Read the model definition and answer for the solid it produces. Units are mm, in the model's axes. A direction names the side the tool comes from. Round coordinates to 2 decimals unless told otherwise and drop trailing zeros. Loops run counter-clockwise (first coordinate to the right, second up) from the corner with the lowest first, then second, coordinate; pieces in that order, holes last. Notation, with made-up numbers: M 59.5,-9.75 L 88.5,-9.75 A9 ccw 88.5,5.25 Z; hole C -34.75,37.5 d4. An arc over 180 degrees is marked long. Write each question's results on one line, items separated by ' | '.
from build123d import *

# Parameters (mm, degrees)
PAD_DEPTH            = 2
PAD001_DEPTH         = 3.5
SKETCH002_R          = 1.5
POCKET_DEPTH         = 5
POCKET001_DEPTH      = 5
LINEARPATTERN_COUNT  = 12
LINEARPATTERN_PITCH  = 4.545455
SKETCH004_W          = 12
SKETCH004_H          = 7.5
POCKET002_DEPTH      = 10
POCKET002_DEPTH_BACK = -100


with BuildPart() as part:
    # Sketch → Pad (new body)
    with BuildSketch(Plane.XY):
        with BuildLine():
            Line((-44.5, 38), (44.5, 38))
            ThreePointArc((49.5, 33), (48.035534, 36.535534), (44.5, 38))
            Line((49.5, 33), (49.5, -33))
            ThreePointArc((44.5, -38), (48.035534, -36.535534), (49.5, -33))
            Line((44.5, -38), (-44.5, -38))
            ThreePointArc((-49.5, -33), (-48.035534, -36.535534), (-44.5, -38))
            Line((-49.5, -33), (-49.5, 33))
            ThreePointArc((-44.5, 38), (-48.035534, 36.535534), (-49.5, 33))
        make_face()
    extrude(amount=PAD_DEPTH)

    # Sketch001 (on Face10 of Pad) → Pad001 (join)
    with BuildSketch(Plane.XY.offset(2)):
        with BuildLine():
            Line((-44.5, 36), (30.5, 36))
            ThreePointArc((33.5, 33), (32.62132, 35.12132), (30.5, 36))
            Line((33.5, 33), (33.5, 25))
            ThreePointArc((33.5, 25), (34.37868, 22.87868), (36.5, 22))
            Line((36.5, 22), (44.5, 22))
            ThreePointArc((47.5, 19), (46.62132, 21.12132), (44.5, 22))
            Line((47.5, 19), (47.5, -33))
            ThreePointArc((44.5, -36), (46.62132, -35.12132), (47.5, -33))
            Line((44.5, -36), (-30.5, -36))
            ThreePointArc((-33.5, -33), (-32.62132, -35.12132), (-30.5, -36))
            Line((-33.5, -33), (-33.5, -25))
            ThreePointArc((-33.5, -25), (-34.37868, -22.87868), (-36.5, -22))
            Line((-36.5, -22), (-44.5, -22))
            ThreePointArc((-47.5, -19), (-46.62132, -21.12132), (-44.5, -22))
            Line((-47.5, -19), (-47.5, 33))
            ThreePointArc((-44.5, 36), (-46.62132, 35.12132), (-47.5, 33))
        make_face()
        with BuildLine():
            Line((-46, -19), (-46, 33))
            ThreePointArc((-44.5, 34.5), (-45.56066, 34.06066), (-46, 33))
            Line((-44.5, 34.5), (30.5, 34.5))
            ThreePointArc((32, 33), (31.56066, 34.06066), (30.5, 34.5))
            Line((32, 33), (32, 25))
            ThreePointArc((32, 25), (33.318019, 21.818019), (36.5, 20.5))
            Line((36.5, 20.5), (44.5, 20.5))
            ThreePointArc((46, 19), (45.56066, 20.06066), (44.5, 20.5))
            Line((46, 19), (46, -33))
            ThreePointArc((44.5, -34.5), (45.56066, -34.06066), (46, -33))
            Line((44.5, -34.5), (-30.5, -34.5))
            ThreePointArc((-32, -33), (-31.56066, -34.06066), (-30.5, -34.5))
            Line((-32, -33), (-32, -25))
            ThreePointArc((-32, -25), (-33.318019, -21.818019), (-36.5, -20.5))
            Line((-36.5, -20.5), (-44.5, -20.5))
            ThreePointArc((-46, -19), (-45.56066, -20.06066), (-44.5, -20.5))
        make_face(mode=Mode.SUBTRACT)
    extrude(amount=-PAD001_DEPTH)

    # Sketch002 (on Face5 of Pad001) → Pocket (cut)
    with BuildSketch(Plane.XY.offset(2)):
        with Locations((40.5, 29)):
            Circle(SKETCH002_R)
        with Locations((-40.5, -29)):
            Circle(SKETCH002_R)
    extrude(amount=-POCKET_DEPTH, mode=Mode.SUBTRACT)

    # Sketch003 (on Face46 of Pocket) → Pocket001 (cut)
    with BuildSketch(Plane.XY.offset(2)):
        with BuildLine():
            ThreePointArc((-24, 20), (-25, 21), (-26, 20))
            Line((-26, 20), (-26, -20))
            ThreePointArc((-26, -20), (-25, -21), (-24, -20))
            Line((-24, 20), (-24, -20))
        make_face()
    pocket001 = extrude(amount=-POCKET001_DEPTH, mode=Mode.SUBTRACT)

    # LinearPattern: Pocket001 ×12
    with Locations(*[(i * LINEARPATTERN_PITCH, 0, 0) for i in range(1, LINEARPATTERN_COUNT)]):
        add(pocket001, mode=Mode.SUBTRACT)

    # Sketch004 (on Face4 of LinearPattern) → Pocket002 (cut, two sides)
    with BuildSketch(Plane(origin=(0, 0, 0), x_dir=(1, 0, 0), z_dir=(0, 0, -1))) as pocket002_sk:
        with Locations((-43.5, -19.75)):
            Rectangle(SKETCH004_W, SKETCH004_H)
    extrude(amount=-POCKET002_DEPTH, mode=Mode.SUBTRACT)
    extrude(pocket002_sk.sketch, amount=-POCKET002_DEPTH_BACK, mode=Mode.SUBTRACT)


solid = part.part
Item 1: The part is cut by section A-A (x = 40.5). Determine the outline of the cut face in (y, z), plus the area to 4 significant figures.
Outcome:
outline: M -38,0 L -36,0 L -36,-1.5 L -34.5,-1.5 L -34.5,0 L 20.5,0 L 20.5,-1.5 L 22,-1.5 L 22,0 L 27.5,0 L 27.5,2 L -38,2 Z; M 30.5,0 L 38,0 L 38,2 L 30.5,2 Z | area: 150.5 mm2
Item 2: For faces 5 (the face through (11.2, -36.4, 0)), 6 (the face through (-5.818, 0, 1)), 7 (the face through (-37.5, 20, 1)), 8 (the face through (34.36, 22.9, -0.74)), determine the directions among +Z, -Z, +X, -X, +Y, -Y from which every point of the face is accessible in a straight line to the end or side of a thin tool.
Outcome:
face 5: -Z | face 6: +Z, -Z | face 7: +Z, -Z, -X | face 8: -Z, +X, +Y
Item 3: Flat-ended cylindrical pins translate along their axes: pin 1 (1.6 mm diameter, centred on y = 19.5, z = 1, fed in from -X); pin 2 (3.5 mm diameter, centred on x = 40.5, y = 29, fed in from -Z); pin 3 (0.8 mm diameter, centred on y = -1, z = -0.5, fed in from -X). Find the tip coordinate at first contact, or state that the pin passes through.
Outcome:
pin 1: stops at x = -37.5 | pin 2: stops at z = 0 | pin 3: stops at x = -47.5
Item 4: The part is cut by section C-C (z = 1.4). State how many separate pieces and enclosed holes the cut face has, plus the area to 3 significant figures.
Outcome:
separate pieces: 1 | enclosed holes: 14 | area: 6,400 mm2
Item 5: Straight lines are drawn through the part: line 1 (Y direction, x = 14.5, z = -0.8); line 2 (X direction, y = 2, z = -0.35); line 3 (Y direction, x = 40.5, z = 1.3). For each, find the intervals that lie inside material, in ascending order.
Outcome:
line 1: y = -36 to -34.5, 34.5 to 36 | line 2: x = -47.5 to -46, 46 to 47.5 | line 3: y = -38 to 27.5, 30.5 to 38
Item 6: The mould has two halves that part along X. Classify faces 1 (the face through (-49.5, -9, 1)), 2 (the face through (-44, 16, 1)), 3 (the face through (49.5, 0, 1)), 4 (the face through (33.283, 21.853, -0.74)): pulls with the +X half, pulls with the -X half, needs draft (parallel to the pull), parting line crosses it, or undercut.
Outcome:
face 1: pulls with the -X half | face 2: needs draft | face 3: pulls with the +X half | face 4: undercut
Item 7: The part is cut by section B-B (y = -29). Determine the outline of the cut face in (x, z).
Outcome:
outline: M -49.5,0 L -42,0 L -42,2 L -49.5,2 Z; M -39,0 L -33.5,0 L -33.5,-1.5 L -32,-1.5 L -32,0 L 46,0 L 46,-1.5 L 47.5,-1.5 L 47.5,0 L 49.5,0 L 49.5,2 L -39,2 Z
